Read the model definition and answer for the solid it produces. Units are mm, in the model's axes. Face numbers are marked on the shaded views. Coordinates: 2 decimals unless noted, no trailing zeros. Write each loop counter-clockwise with the first axis right and the second up, starting at its lowest first coordinate (ties: lowest second). Pieces come first, ordered by that corner, then holes.
1) Find the intervals of material crossed by line 1 (Z direction, x = 2, y = -2.75); line 2 (X direction, y = -3.25, z = 10.25); line 3 (Y direction, x = 3, z = 16.25), in increasing order.
2) The part is cut by section B-B (z = 11.25). Determine the outline of the cut face in (x, y), then the cut area to 3 significant figures.
3) The part is cut by section D-D (x = -31.5). Determine the outline of the cut face in (y, z), then the cut area to 3 significant figures.
4) Determine the mould class of the marked faces 1, 2 and 3 for opening direction X: +X half, -X half, draft (parallel to the pull), parting line (faces both ways), or undercut.
5) The part is cut by section C-C (x = -5). Determine the outline of the cut face in (y, z), then the cut area to 3 significant figures.
6) The part is cut by section A-A (y = -4.5). Determine the outline of the cut face in (x, z).
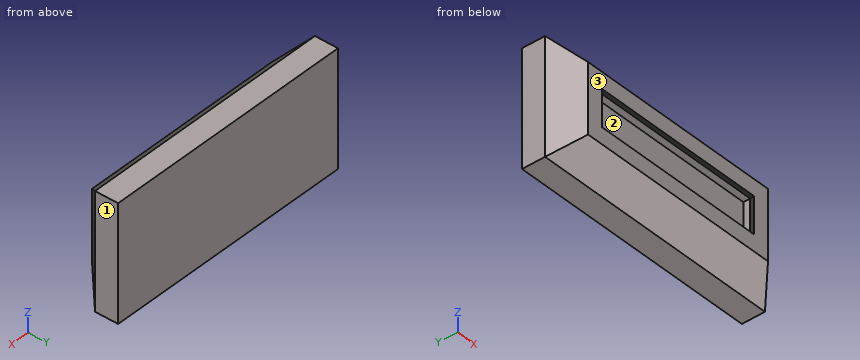
from build123d import *

# Parameters (mm, degrees)
F0_W     = 55
F0_H     = 25
F1_DEPTH = 10
F2_SIZE  = 5
F3_T     = -2.5


with BuildPart() as f1:
    # F0 (on Front) → F1 (new body)
    with BuildSketch(Plane.XZ):
        with Locations((-10.534275, 17.852823)):
            Rectangle(F0_W, F0_H)
    extrude(amount=F1_DEPTH)

    # F2
    f2_edges = [f1.edges().sort_by_distance(p)[0] for p in [
        (-10.534275, -10, 30.352823),
        (-38.034275, -10, 17.852823),
        (-10.534275, -10, 5.352823),
        (16.965725, -10, 17.852823),
    ]]
    chamfer(f2_edges, length=F2_SIZE)

    # F3
    f3_openings = [f1.faces().sort_by_distance(p)[0] for p in [
        (-10.534275, -10, 17.852823),
    ]]
    offset(amount=F3_T, openings=f3_openings)


solid = f1.part
Reported:
1. line 1: z = 5.35 to 7.85, 27.85 to 30.35
1. line 2: x = -38.03 to -35.53, 14.47 to 16.97
1. line 3: y = -2.5 to 0
2. outline: (-38.03, -5) - (-33.03, -10) - (11.97, -10) - (16.97, -5) - (16.97, 0) - (-38.03, 0) - close; hole (-35.53, -3.96) - (-32.14, -7.36) - (11.07, -7.36) - (14.47, -3.96) - (14.47, -2.5) - (-35.53, -2.5) - close
2. area: 293 mm2
3. outline: (-10, 10.35) - (-5, 5.35) - (0, 5.35) - (0, 30.35) - (-5, 30.35) - (-10, 25.35) - close; hole (-8, 11.89) - (-3.96, 7.85) - (-2.5, 7.85) - (-2.5, 27.85) - (-3.96, 27.85) - (-8, 23.82) - close
3. area: 131 mm2
4. face 1: +X half
4. face 2: undercut
4. face 3: draft
5. outline: (-10, 10.35) - (-5, 5.35) - (0, 5.35) - (0, 30.35) - (-5, 30.35) - (-10, 25.35) - (-10, 21.82) - (-3.96, 27.85) - (-2.5, 27.85) - (-2.5, 7.85) - (-3.96, 7.85) - (-10, 13.89) - close
5. area: 111 mm2
6. outline: (-38.03, 5.35) - (16.97, 5.35) - (16.97, 30.35) - (-38.03, 30.35) - close; hole (-35, 8.39) - (13.93, 8.39) - (13.93, 27.32) - (-35, 27.32) - close
